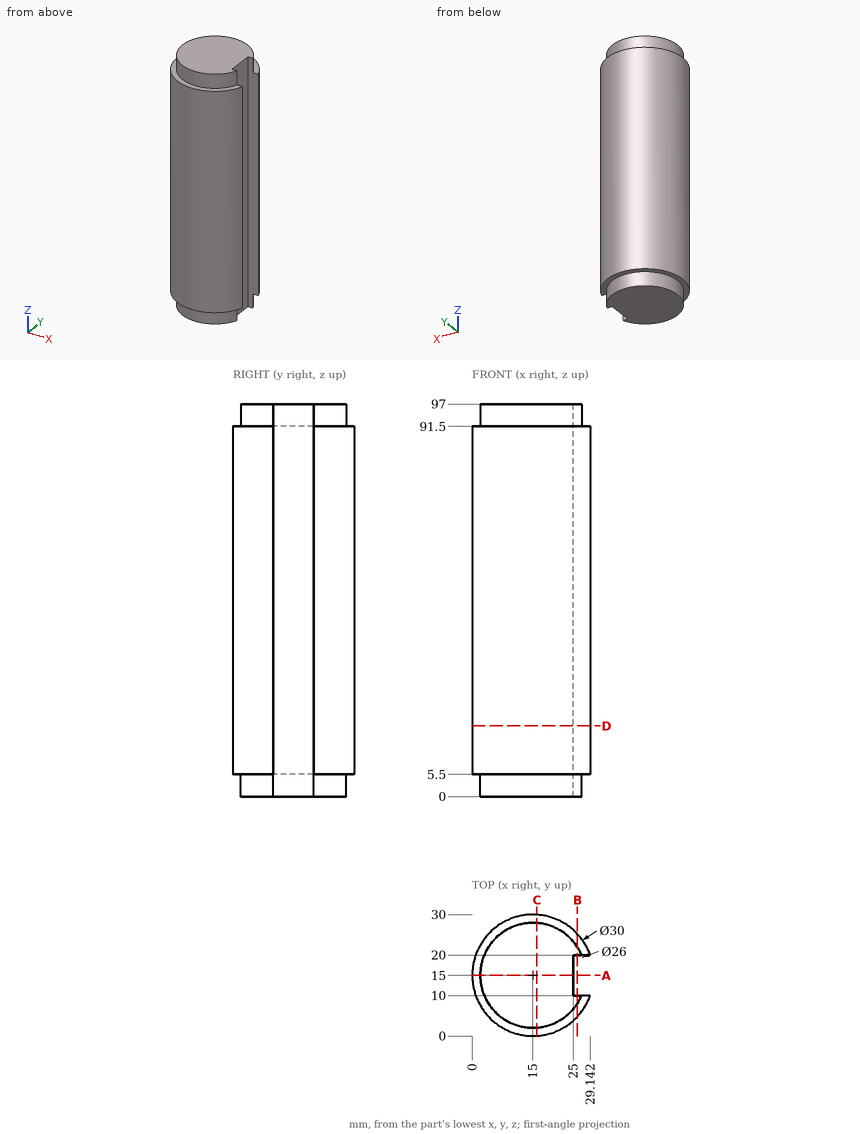
Answer from the drawing. Dimensions are ordinates in mm from the lowest x, y and z of the part. Give positions to 0.01 mm unless a question says otherwise; leave off trailing zeros. Loops run counter-clockwise (first coordinate to the right, second up) from the corner with the lowest first, then second, coordinate; pieces in that order, holes last. Notation, with made-up numbers: (2, 88.25) -> (22, 88.25) arc R13 ccw to (22, 106.25) -> close; hole circle Ø8 at (75.25, 30.25). An arc over 180 degrees is marked (long way). Use a Markdown table: item, result.
Q1. Section D-D, the plane z = 17.5 is taken. Determine the outline of the cut face in (x, y), then the cut area to 3 significant figures.
Solved:
| item | result |
|---|---|
| outline | (25, 10) -> (25, 20) -> (29.14, 20) arc R15 ccw (long way) to (29.14, 10) -> close |
| area | 660 mm^2 |
Q2. Section B-B, the plane x = 26 is taken. Determine the outline of the cut face in (y, z).
Solved:
| item | result |
|---|---|
| outline | (4.8, 5.5) -> (8.07, 5.5) -> (8.07, 0) -> (10, 0) -> (10, 97) -> (8.07, 97) -> (8.07, 91.5) -> (4.8, 91.5) -> close; (20, 0) -> (21.93, 0) -> (21.93, 5.5) -> (25.2, 5.5) -> (25.2, 91.5) -> (21.93, 91.5) -> (21.93, 97) -> (20, 97) -> close |
Q3. Section C-C, the plane x = 16 is taken. Determine the outline of the cut face in (y, z), then the cut area to 3 significant figures.
Solved:
| item | result |
|---|---|
| outline | (0.03, 5.5) -> (2.04, 5.5) -> (2.04, 0) -> (27.96, 0) -> (27.96, 5.5) -> (29.97, 5.5) -> (29.97, 91.5) -> (27.96, 91.5) -> (27.96, 97) -> (2.04, 97) -> (2.04, 91.5) -> (0.03, 91.5) -> close |
| area | 2,860 mm^2 |
Q4. Each of these flat-tipped pins is pushed along its axis until it touches: pin 1 (5 mm diameter, centred on y = 13.5, z = 57, fed in from +X); pin 2 (5 mm diameter, centred on y = 19.5, z = 71, fed in from -X); pin 3 (4.5 mm diameter, centred on x = 26.5, z = 66, fed in from +Y). Where does it stop, or does it pass through?
Solved:
| item | result |
|---|---|
| pin 1 | stops at x = 25 |
| pin 2 | stops at x = 0.13 |
| pin 3 | stops at y = 26.81 |
Q5. Section A-A, the plane y = 15 is taken. Determine the outline of the cut face in (x, z), then the cut area to 3 significant figures.
Solved:
| item | result |
|---|---|
| outline | (0, 5.5) -> (2, 5.5) -> (2, 0) -> (25, 0) -> (25, 97) -> (2, 97) -> (2, 91.5) -> (0, 91.5) -> close |
| area | 2,400 mm^2 |
Q6. Find the intervals of material crossed by line 1 along Y through (x, z) = (7.5, 8); line 2 along Y through (x, z) = (14.25, 23), in increasing order.
Solved:
| item | result |
|---|---|
| line 1 | y = 2.01 to 27.99 |
| line 2 | y = 0.02 to 29.98 |
